```python
from build123d import *


with BuildPart() as part:
    # Sketch1 → Revolve1 (revolve)
    with BuildSketch(Plane.XY):
        Polygon((-17, 0), (-17, 3.233), (-16.233, 4), (0, 4), (0, 0), align=None)
    revolve(axis=Axis((0, 0, 0), (-1, 0, 0)))

    # Sketch2 → Revolve2 (revolve)
    with BuildSketch(Plane.XY):
        with BuildLine():
            Line((0, 0), (0, 6.5))
            Line((0, 6.5), (8, 6.5))
            ThreePointArc((8, 6.5), (12.371375393, 4.81051735), (14.470331437, 0.620331437))
            Line((14.470331437, 0.620331437), (13.85, 0))
            Line((13.85, 0), (0, 0))
        make_face()
    revolve(axis=Axis((50, 0, 0), (-1, 0, 0)))

    # Sketch3 → Cut-Revolve1 (revolve, cut)
    with BuildSketch(Plane.XY):
        with BuildLine():
            Line((-0.826794919, 3.9), (-0.173205081, 3.9))
            ThreePointArc((-0.173205081, 3.9), (-0.073205081, 3.926794919), (0, 4))
            Line((0, 4), (0, 4.9))
            Line((0, 4.9), (-1, 4.9))
            Line((-1, 4.9), (-1, 4))
            ThreePointArc((-1, 4), (-0.926794919, 3.926794919), (-0.826794919, 3.9))
        make_face()
    revolve(axis=Axis((0, 0, 0), (-1, 0, 0)), mode=Mode.SUBTRACT)


solid = part.part
```
Part model, mm, in its own coordinate system. A direction names the side the tool comes from. Round coordinates to 2 decimals unless told otherwise and drop trailing zeros. Loops run counter-clockwise (first coordinate to the right, second up) from the corner with the lowest first, then second, coordinate; pieces in that order, holes last. Notation, with made-up numbers: (-22, -13) -> (31, -13) arc R28 cw to (31, 7) -> close; hole circle Ø8 at (33.25, 57). An arc over 180 degrees is marked (long way). Use CSV: the item, a comma, the result in double quotes. Start each with the question number.
1) Cut at C-C, the plane x = -13. Write the cut outline in (y, z), plus the area to 3 significant figures.
2) Which spindle directions (+Z, -Z, +X, -X, +Y, -Y) get a long thin tool onto all of the face, cutting with end or side? Do faces 4 (the cylindrical face through (-8.51, -0.867, 3.905)), 5 (the flat face through (-17, 0, 0)). Say none if no direction does.
3) Drop flat-ended pins along their axis: P1, Ø1.5, axis at x = -13, z = 0, coming from the -Y side; P2, Ø1.5, axis at x = -6, z = 3.5, coming from the -Y side; P3, Ø5, axis at x = -13.5, z = 0, coming from the +Y side. Give the stop position or say it passes through.
4) Wall check: L1, parallel to Y at x = 4, z = 0.25; L2, parallel to Z at x = 13, y = -3; L3, parallel to Z at x = 5.5, y = -1.5. Give the ranges that are in metal, low to high. Write a range as [from, to].
5) Cut at A-A, the plane x = 10.5. Write the cut outline in (y, z), plus the area to 3 significant figures.
6) Cut at B-B, the plane y = 4.5. Write the cut outline in (x, z).
7) Pull direction X, two halves, no side cores. Call faces 1 (the cylindrical face through (4.056, -5.158, 3.955)), 2 (the cylindrical face through (-0.5, -2.87, -2.64)), 3 (the flat face through (0, -3, -3)): +X half, -X half, draft (parallel to the pull), parting line (faces both ways), or undercut.
Determined:
1,outline,"circle Ø8 at (0, 0)"
1,area,"50.3 mm2"
2,face 4,"-X"
2,face 5,"+Z, -Z, -X, +Y, -Y"
3,P1,"stops at y = -4"
3,P2,"stops at y = -2.9"
3,P3,"stops at y = 4"
4,L1,"y = [-6.5, 6.5]"
4,L2,"z = [-2.87, 2.87]"
4,L3,"z = [-6.32, 6.32]"
5,outline,"circle Ø12 at (0, 0)"
5,area,"113 mm2"
6,outline,"(0, -4.69) -> (8, -4.69) arc R4.69 ccw to (8, 4.69) -> (0, 4.69) -> close"
7,face 1,"draft"
7,face 2,"undercut"
7,face 3,"-X half"
